Verification items for the finished model (mm, model axes). A direction names the side the tool comes from. Round coordinates to 2 decimals unless told otherwise and drop trailing zeros. Write each loop counter-clockwise with the first axis right and the second up, starting at its lowest first coordinate (ties: lowest second). Pieces come first, ordered by that corner, then holes. Notation, with made-up numbers: (-21, 0) - (2, 0) arc R12 ccw to (2, 15) - close; hole circle Ø9 at (26.25, 44.5). An arc over 180 degrees is marked (long way). Answer as a JSON object with one key per item and string values.
```python
from build123d import *

# Parameters (mm, degrees)
BARRER1_PROFILE_R       = 16
CROQUIS22_W             = 24
CROQUIS22_H             = 30
CROQUIS22_R             = 5.5
SALIENTE_EXTRUIR1_DEPTH = 3
CROQUIS23_R             = 12.5
SALIENTE_EXTRUIR2_DEPTH = 24
SALIENTE_EXTRUIR2_TAPER = 0.1
REDONDEO1_R             = 2
REDONDEO2_R             = 2


with BuildPart() as part:
    # Barrer1: sweep along a curve in space
    with BuildLine() as barrer1_path:
        Line((1184.694036121, -317.266225222, 2234.993228397), (1184.694036121, -961.667575773, 2234.993228397))
        ThreePointArc((1184.694036121, -961.667575773, 2234.993228397), (1184.694036121, -1060.66252514, 2275.998279031), (1184.694036121, -1101.667575773, 2374.993228397))
        Line((1184.694036121, -1101.667575773, 2374.993228397), (1184.694036121, -1101.667575773, 3598.952990458))
    # Barrer1 profile (on start of the path) → Barrer1 (sweep)
    with BuildSketch(Plane(origin=(1184.694036121, -317.266225222, 2234.993228397), x_dir=(0, 0, -1), z_dir=(0, -1, 0))):
        Circle(BARRER1_PROFILE_R)
    sweep(path=barrer1_path.line)



with BuildPart() as body_2:
    # Croquis22 → Saliente-Extruir1 (new body)
    with BuildSketch(Plane.XY.offset(2234.993228397)):
        with Locations((1184.694036121, -279.321290843)):
            Rectangle(CROQUIS22_W, CROQUIS22_H)
        with Locations((1184.694036121, -273.810487485)):
            Circle(CROQUIS22_R, mode=Mode.SUBTRACT)
    extrude(amount=SALIENTE_EXTRUIR1_DEPTH)


with BuildPart() as part_1:
    add(part.part)

    add(body_2.part)  # Saliente-Extruir2 merges body 2
    # Croquis23 → Saliente-Extruir2 (add)
    with BuildSketch(Plane(origin=(0, -317.266225222, 0), x_dir=(1, 0, 0), z_dir=(0, 1, 0))):
        with Locations((1184.694036121, -2234.993228397)):
            Circle(CROQUIS23_R)
    extrude(amount=SALIENTE_EXTRUIR2_DEPTH, taper=SALIENTE_EXTRUIR2_TAPER)

    # Redondeo1
    # the kernel refuses this fillet: 2 mm, written as the material it takes off along each edge
    with BuildSketch(Plane(origin=(1184.694036121, -293.266225222, 2234.993228397), x_dir=(1, 0, 0), z_dir=(0, 0, -1))) as redondeo1_piece_1_section:
        with BuildLine():
            CenterArc((12.458112055 - REDONDEO1_R * 0.998256192065, REDONDEO1_R), REDONDEO1_R, 270, 89.9)
            Line((12.458112055 - REDONDEO1_R * 0.998256192065, 0), (12.458112055, 0))
            Line((12.458112055, 0), (12.458112055 + REDONDEO1_R * 0.00174228484855, REDONDEO1_R * 0.998254671634))
        make_face()
    redondeo1_piece_1 = revolve(axis=Axis((1184.694036121, -293.266225222, 2234.993228397), (0, -1, 0)), mode=Mode.PRIVATE)
    redondeo1_piece_1 = split(redondeo1_piece_1, bisect_by=Plane(origin=(1196.694036121, -293.909040816, 2236.28595065), z_dir=(1, 0, 0)), keep=Keep.TOP, mode=Mode.PRIVATE)
    add(redondeo1_piece_1, mode=Mode.SUBTRACT)
    with BuildSketch(Plane(origin=(1184.694036121, -293.266225222, 2234.993228397), x_dir=(1, 0, 0), z_dir=(0, 0, -1))) as redondeo1_piece_2_section:
        with BuildLine():
            CenterArc((12.458112055 - REDONDEO1_R * 0.998256192065, REDONDEO1_R), REDONDEO1_R, 270, 89.9)
            Line((12.458112055 - REDONDEO1_R * 0.998256192065, 0), (12.458112055, 0))
            Line((12.458112055, 0), (12.458112055 + REDONDEO1_R * 0.00174228484855, REDONDEO1_R * 0.998254671634))
        make_face()
    redondeo1_piece_2 = revolve(axis=Axis((1184.694036121, -293.266225222, 2234.993228397), (0, -1, 0)), mode=Mode.PRIVATE)
    redondeo1_piece_2 = split(redondeo1_piece_2, bisect_by=Plane(origin=(1184.694036121, -293.82884964, 2234.993228397), z_dir=(0, 0, -1)), keep=Keep.TOP, mode=Mode.PRIVATE)
    add(redondeo1_piece_2, mode=Mode.SUBTRACT)
    with BuildSketch(Plane(origin=(1184.694036121, -293.266225222, 2234.993228397), x_dir=(1, 0, 0), z_dir=(0, 0, -1))) as redondeo1_piece_3_section:
        with BuildLine():
            CenterArc((12.458112055 - REDONDEO1_R * 0.998256192065, REDONDEO1_R), REDONDEO1_R, 270, 89.9)
            Line((12.458112055 - REDONDEO1_R * 0.998256192065, 0), (12.458112055, 0))
            Line((12.458112055, 0), (12.458112055 + REDONDEO1_R * 0.00174228484855, REDONDEO1_R * 0.998254671634))
        make_face()
    redondeo1_piece_3 = revolve(axis=Axis((1184.694036121, -293.266225222, 2234.993228397), (0, -1, 0)), mode=Mode.PRIVATE)
    redondeo1_piece_3 = split(redondeo1_piece_3, bisect_by=Plane(origin=(1184.694036121, -293.82954, 2237.993228397), z_dir=(0, 0, 1)), keep=Keep.TOP, mode=Mode.PRIVATE)
    add(redondeo1_piece_3, mode=Mode.SUBTRACT)
    with BuildSketch(Plane(origin=(1184.694036121, -293.266225222, 2234.993228397), x_dir=(1, 0, 0), z_dir=(0, 0, -1))) as redondeo1_piece_4_section:
        with BuildLine():
            CenterArc((12.458112055 - REDONDEO1_R * 0.998256192065, REDONDEO1_R), REDONDEO1_R, 270, 89.9)
            Line((12.458112055 - REDONDEO1_R * 0.998256192065, 0), (12.458112055, 0))
            Line((12.458112055, 0), (12.458112055 + REDONDEO1_R * 0.00174228484855, REDONDEO1_R * 0.998254671634))
        make_face()
    redondeo1_piece_4 = revolve(axis=Axis((1184.694036121, -293.266225222, 2234.993228397), (0, -1, 0)), mode=Mode.PRIVATE)
    redondeo1_piece_4 = split(redondeo1_piece_4, bisect_by=Plane(origin=(1172.694036121, -293.908477317, 2236.286131644), z_dir=(-1, 0, 0)), keep=Keep.TOP, mode=Mode.PRIVATE)
    add(redondeo1_piece_4, mode=Mode.SUBTRACT)

    # Redondeo2
    redondeo2_edges = [part_1.edges().sort_by_distance(p)[0] for p in [
        (1184.694036121, -317.266225222, 2250.993228397),
    ]]
    fillet(redondeo2_edges, radius=REDONDEO2_R)


solid = part_1.part
```
1. Cross-section at A-A (z = 3148). Record the boundary of the cut face in (x, y).
Completed:
{"outline": "circle Ø32 at (1184.69, -1101.67)"}
2. Material ranges on probe 1 along Z at (x, y) = (1175, -869); probe 2 along Y at (x, z) = (1187, 2533); probe 3 along Z at (x, y) = (1182.5, -622), recorded low to high. Write a range as from..to.
Completed:
{"probe 1": "z = 2222.26..2247.72", "probe 2": "y = -1117.5..-1085.83", "probe 3": "z = 2219.14..2250.84"}
3. Cross-section at B-B (y = -349.5). Record the boundary of the cut face in (x, z).
Completed:
{"outline": "circle Ø32 at (1184.69, 2234.99)"}
4. Access from +Z, -Z, +X, -X, +Y, -Y to the whole of each face (thin tool, end or side, straight path). Record for faces 1 (the face through (1178.57, -1116.45, 2995.54)), 2 (the face through (1196.598, -306.11, 2231.244)), 3 (the face through (1184, -1101, 3598.953)).
Completed:
{"face 1": "+Z", "face 2": "+Y", "face 3": "+Z, +X, -X, +Y, -Y"}
5. Go/stop test with flat-tipped pins: pin 1 (6 mm diameter, centred on x = 1179, y = -998.5, fed in from +Z); pin 2 (6 mm diameter, centred on x = 1190, y = -815.5, fed in from -Z); pin 3 (3.5 mm diameter, centred on y = -284, z = 2236, fed in from -X). Record where each tip stops, or that it passes through.
Completed:
{"pin 1": "stops at z = 2256.86", "pin 2": "stops at z = 2219.16", "pin 3": "stops at x = 1172.69"}
